Here's how the part is built. I have some questions about the finished solid (model axes, mm). A direction names the side the tool comes from. Give positions to 0.01 mm unless a question says otherwise; leave off trailing zeros. Write each loop counter-clockwise with the first axis right and the second up, starting at its lowest first coordinate (ties: lowest second). Pieces come first, ordered by that corner, then holes. Notation, with made-up numbers: (21.5, 87.25) - (25.5, 87.25) arc R21 ccw to (25.5, 121.25) - close; hole circle Ø8 at (40.25, -36.5). An arc over 180 degrees is marked (long way). One line per item, written item: value. Start each with the question number.
1) We'd pull the mould along Z, two halves only. Please class faces 6 (the flat face through (-182.744, 139.865, 141.627)), 7 (the flat face through (117.401, -107, 0)), 8 (the conical face through (-83.5, -369.02, 3.42)): +Z half, -Z half, draft (parallel to the pull), parting line (faces both ways), or undercut.
2) Please list where these lines run through material, in increasing order: L1, parallel to Y at x = 341, z = 17; L2, parallel to Y at x = -84.5, z = -176; L3, parallel to X at y = -274, z = -56. Write a range as [from, to].
3) Imagine slicing it at D-D on y = 117.5. Write out the boundary of the cut face in (x, z).
4) On a 3-axis mill with a long thin cutter (end or side, diameter ignored), from which of +Z, -Z, +X, -X, +Y, -Y can I reach the whole of each face in a straight line? I mean faces 1 (the cylindrical face through (-102.52, -106.63, 3.97)), 2 (the flat face through (96.803, -360.135, -19.86)), 3 (the flat face through (97.372, -360.135, 19.86)), 4 (the flat face through (210.126, 139.865, 85.197)), 5 (the flat face through (-35.178, 139.865, -226.824)). Say none if no direction works.
5) Imagine slicing it at C-C on z = 263. Write out the boundary of the cut face in (x, y).
6) Imagine slicing it at A-A on x = -155. Write out the boundary of the cut face in (y, z), plus the area to 3 significant figures.
7) Imagine slicing it at B-B on y = 199. Write out the boundary of the cut face in (x, z), plus the area to 3 significant figures.
8) I'm going to push flat-ended pins straight in: P1, Ø4, axis at x = 175, y = 126.5, coming from the -Z side; P2, Ø7.5, axis at x = 102.5, y = -134, coming from the +Z side; P3, Ø19.5, axis at x = 107, y = -47.5, coming from the -Z side; P4, Ø4, axis at x = 233.5, z = 6, coming from the +Y side. Where does each tip first touch, or does it pass through?
from build123d import *
from build123d.topology import SkipClean

# Parameters (mm, degrees)
SKETCH2_R             = 5
BOSS_EXTRUDE2_DEPTH   = 18
BOSS_EXTRUDE2_2_DEPTH = 18
BOSS_EXTRUDE2_3_DEPTH = 18
BOSS_EXTRUDE3_START   = -2
BOSS_EXTRUDE3_DEPTH   = 2
BOSS_EXTRUDE4_DEPTH   = 50
CHAMFER5_SIZE         = 2
SCALE1_SCALE          = 10


with BuildPart() as part:
    # Sketch2 → Boss-Extrude2 (new body)
    with BuildSketch(Plane(origin=(0, 0, 0), x_dir=(1, 0, 0), z_dir=(0, 1, 0))):
        with Locations(Location((33.75, 0, 0), (0, 0, 270))):
            Circle(SKETCH2_R)
    extrude(amount=BOSS_EXTRUDE2_DEPTH)



with BuildPart() as body_2:
    # Sketch2 → Boss-Extrude2 2 (new body)
    with BuildSketch(Plane(origin=(0, 0, 0), x_dir=(1, 0, 0), z_dir=(0, 1, 0))):
        with Locations(Location((-16.875, -29.228357378, 0), (0, 0, 270))):
            Circle(SKETCH2_R)
    extrude(amount=BOSS_EXTRUDE2_2_DEPTH)


with BuildPart() as body_3:
    # Sketch2 → Boss-Extrude2 3 (new body)
    with BuildSketch(Plane(origin=(0, 0, 0), x_dir=(1, 0, 0), z_dir=(0, 1, 0))):
        with Locations(Location((-16.875, 29.228357378, 0), (0, 0, 270))):
            Circle(SKETCH2_R)
    extrude(amount=BOSS_EXTRUDE2_3_DEPTH)


with BuildPart() as part_1:
    with SkipClean():  # the faces are left unmerged after this step: merging them gives an invalid solid
        add(part.part)

        add(body_2.part)  # Boss-Extrude3 merges body 2

        add(body_3.part)  # Boss-Extrude3 merges body 3
        # Sketch5 → Boss-Extrude3 (add)
        with BuildSketch(Plane(origin=(0, 0, 0), x_dir=(1, 0, 0), z_dir=(0, 1, 0)).offset(BOSS_EXTRUDE3_START)):
            with BuildLine():
                Line((-13.339466094, 32.763891284), (7.109833073, 12.314592116))
                Line((7.109833073, 12.314592116), (35.044095226, 4.829629131))
                ThreePointArc((35.044095226, 4.829629131), (38.75, 0), (35.044095226, -4.829629131))
                Line((35.044095226, -4.829629131), (7.109833073, -12.314592116))
                Line((7.109833073, -12.314592116), (-13.339466094, -32.763891284))
                ThreePointArc((-13.339466094, -32.763891284), (-19.375, -33.558484397), (-21.704629131, -27.934262152))
                Line((-21.704629131, -27.934262152), (-14.219666147, 0))
                Line((-14.219666147, 0), (-21.704629131, 27.934262152))
                ThreePointArc((-21.704629131, 27.934262152), (-19.375, 33.558484397), (-13.339466094, 32.763891284))
            make_face()
        extrude(amount=BOSS_EXTRUDE3_DEPTH)

    # Sketch6 → Boss-Extrude4 (add)
    with SkipClean():  # the faces are left unmerged after this step: merging them gives an invalid solid
        with BuildSketch(Plane.XZ.offset(2)):
            with BuildLine():
                Line((9.539392014, -3), (12, -3))
                Line((12, -3), (12, 3))
                Line((12, 3), (9.539392014, 3))
                ThreePointArc((9.539392014, 3), (-10, 0), (9.539392014, -3))
            make_face()
        extrude(amount=BOSS_EXTRUDE4_DEPTH)

    # Chamfer5
    chamfer5_edges = [part_1.edges().sort_by_distance(p)[0] for p in [
        (12, -52, 0),
        (10.769696007, -52, 3),
        (-10, -52, 0),
        (10.769696007, -52, -3),
    ]]
    chamfer(chamfer5_edges, length=CHAMFER5_SIZE)


with BuildPart() as part_2:
    # Scale1: scaled about (0.288742854, -16.667261458, 0)
    add(part_1.part.scale(SCALE1_SCALE).moved(Location((-2.598685686, 150.005353122, 0))))


solid = part_2.part
Numbers:
1. face 6: undercut
1. face 7: draft
1. face 8: parting line
2. L1: [130.01, 330.01]
2. L2: [130.01, 150.01]
2. L3: [-85.45, 80.25]
3. outline: (92.8, -30) - (117.4, -30) - (117.4, 30) - (92.8, 30) arc R100 ccw (long way) to start
4. face 1: -Y
4. face 2: -Z, +X, -Y
4. face 3: +Z, +X, -Y
4. face 4: +Z, +X, +Y, -Y
4. face 5: -Z, +X, +Y, -Y
5. outline: (-215.27, 130.01) - (-71.35, 130.01) - (-71.35, 150.01) - (-130.82, 150.01) - (-130.82, 330.01) - (-211.88, 330.01) - (-211.88, 150.01) - (-215.27, 150.01) - close
6. outline: (130.01, -339.54) - (330.01, -339.54) - (330.01, -245.03) - (150.01, -245.03) - (150.01, -38.08) - (130.01, -38.08) - close; (130.01, 38.08) - (150.01, 38.08) - (150.01, 245.03) - (330.01, 245.03) - (330.01, 339.54) - (130.01, 339.54) - close
6. area: 46,100 mm^2
7. outline: circle Ø100 at (-171.35, -292.28); circle Ø100 at (-171.35, 292.28); circle Ø100 at (334.9, 0)
7. area: 23,600 mm^2
8. P1: through
8. P2: z = 30
8. P3: z = -30
8. P4: y = 150.01
